Verification items for the finished model (mm, model axes). A direction names the side the tool comes from. Give positions to 0.01 mm unless a question says otherwise; leave off trailing zeros. Order: outer loops, then holes, each group sorted by start corner. A loop starts at its lowest first (then second) coordinate and runs counter-clockwise, first axis right, second up. Notation, with made-up numbers: (65, -35.5) - (77, -35.5) arc R19 cw to (77, -5.5) - close; hole circle Ø5 at (-19, 77). An arc over 180 degrees is marked (long way). Answer as a JSON object with one key per item and string values.
```python
from build123d import *

# Parameters (mm, degrees)
SKETCH_1_W          = 34
SKETCH_1_H          = 20
SKETCH_1_W_2        = 3
SKETCH_1_H_2        = 12
SKETCH_1_W_3        = 10
SKETCH_1_H_3        = 3
EXTRUDE_1_DEPTH     = 3
SKETCH_2_W          = 2.8
SKETCH_2_H          = 3.3
SKETCH_2_W_2        = 3.2
SKETCH_2_H_2        = 1.35
SKETCH_2_W_3        = 6
CUT_EXTRUDE_1_DEPTH = 3
SKETCH_4_W          = 20
SKETCH_4_H          = 20
SKETCH_4_W_2        = 10
SKETCH_4_H_2        = 3
EXTRUDE_2_DEPTH     = 3
SKETCH_5_W          = 3.2
SKETCH_5_H          = 2.8
SKETCH_5_W_2        = 1.4
SKETCH_5_H_2        = 3.2
SKETCH_5_H_3        = 6
SKETCH_5_W_3        = 1.35
SKETCH_5_W_4        = 3.3
CUT_EXTRUDE_2_DEPTH = 3


with BuildPart() as part:
    # 草图1 → 凸台-拉伸1 (new body)
    with BuildSketch(Plane(origin=(0, 0, 0), x_dir=(1, 0, 0), z_dir=(0, 1, 0))):
        Rectangle(SKETCH_1_W, SKETCH_1_H)
        with Locations((18.5, 0)):
            Rectangle(SKETCH_1_W_2, SKETCH_1_H_2)
        with Locations((0, 11.5)):
            Rectangle(SKETCH_1_W_3, SKETCH_1_H_3)
        with Locations((0, -11.5)):
            Rectangle(SKETCH_1_W_3, SKETCH_1_H_3)
    extrude(amount=EXTRUDE_1_DEPTH)

    # 草图2 → 切除-拉伸1 (cut)
    with BuildSketch(Plane(origin=(0, 3, 0), x_dir=(1, 0, 0), z_dir=(0, 1, 0))):
        with Locations((9.4, 0)):
            Rectangle(SKETCH_2_W, SKETCH_2_H)
        with Locations((12.4, 2.325)):
            Rectangle(SKETCH_2_W_2, SKETCH_2_H_2)
        with Locations((12.4, 0)):
            Rectangle(SKETCH_2_W_2, SKETCH_2_H)
        with Locations((12.4, -2.325)):
            Rectangle(SKETCH_2_W_2, SKETCH_2_H_2)
        with Locations((17, 0)):
            Rectangle(SKETCH_2_W_3, SKETCH_2_H)
    extrude(amount=-CUT_EXTRUDE_1_DEPTH, mode=Mode.SUBTRACT)

    # 草图4 → 凸台-拉伸2 (add)
    with BuildSketch(Plane(origin=(0, 3, 0), x_dir=(1, 0, 0), z_dir=(0, 1, 0))):
        with Locations((-27, 0)):
            Rectangle(SKETCH_4_W, SKETCH_4_H)
        with Locations((-24.6, 11.5)):
            Rectangle(SKETCH_4_W_2, SKETCH_4_H_2)
        with Locations((-24.6, -11.5)):
            Rectangle(SKETCH_4_W_2, SKETCH_4_H_2)
    extrude(amount=-EXTRUDE_2_DEPTH)

    # 草图5 → 切除-拉伸2 (cut)
    with BuildSketch(Plane(origin=(0, 3, 0), x_dir=(1, 0, 0), z_dir=(0, 1, 0))):
        with Locations((0, 2.4)):
            Rectangle(SKETCH_5_W, SKETCH_5_H)
        with Locations((-2.3, 5.4)):
            Rectangle(SKETCH_5_W_2, SKETCH_5_H_2)
        with Locations((0, 10)):
            Rectangle(SKETCH_5_W, SKETCH_5_H_3)
        with Locations((0, 5.4)):
            Rectangle(SKETCH_5_W, SKETCH_5_H_2)
        with Locations((2.3, 5.4)):
            Rectangle(SKETCH_5_W_2, SKETCH_5_H_2)
        with Locations((-26.925, -5.4)):
            Rectangle(SKETCH_5_W_3, SKETCH_5_H_2)
        with Locations((-24.6, -2.4)):
            Rectangle(SKETCH_5_W_4, SKETCH_5_H)
        with Locations((-22.275, -5.4)):
            Rectangle(SKETCH_5_W_3, SKETCH_5_H_2)
        with Locations((-24.6, -5.4)):
            Rectangle(SKETCH_5_W_4, SKETCH_5_H_2)
        with Locations((-24.6, -10)):
            Rectangle(SKETCH_5_W_4, SKETCH_5_H_3)
    extrude(amount=-CUT_EXTRUDE_2_DEPTH, mode=Mode.SUBTRACT)


solid = part.part
```
(1) Access from +Z, -Z, +X, -X, +Y, -Y to the whole of each face (thin tool, end or side, straight path). Record for faces 5 (the flat face through (-33, 2, -10)), 6 (the flat face through (11, 1, 10)), 7 (the flat face through (-19.6, 2, 12)), 8 (the flat face through (10.8, 2, 2)).
Computed values:
{"face 5": "-Z, -X, +Y, -Y", "face 6": "+Z, +X, +Y, -Y", "face 7": "+Z, +Y, -Y", "face 8": "+Y, -Y"}
(2) Release check for a two-part mould opening along Z. For faces 1 (the flat face through (10.8, 2, -2)), 2 (the flat face through (-28, 2, 13)), 3 (the flat face through (1.6, 2, -2)), 4 (the flat face through (-3, 1, -13)) record: pulls with the +Z half, pulls with the -Z half, needs draft (parallel to the pull), parting line crosses it, or undercut.
Computed values:
{"face 1": "undercut", "face 2": "pulls with the +Z half", "face 3": "needs draft", "face 4": "pulls with the -Z half"}
(3) Section check A-A (z = -9). Record the cut outline in (x, y).
Computed values:
{"outline": "(-37, 0) - (-1.6, 0) - (-1.6, 3) - (-37, 3) - close; (1.6, 0) - (17, 0) - (17, 3) - (1.6, 3) - close"}
(4) Material ranges on line 1 along X through (y, z) = (1.05, 2.25); line 2 along X through (y, z) = (0.7, 10.75); line 3 along X through (y, z) = (1.15, 3.25), recorded low to high. Write a range as [from, to].
Computed values:
{"line 1": "x = [-37, -26.25], [-22.95, 10.8], [14, 20]", "line 2": "x = [-29.6, -26.25], [-22.95, -19.6], [-5, 5]", "line 3": "x = [-37, -26.25], [-22.95, 20]"}
(5) Section check B-B (x = 0.5). Record the cut outline in (y, z), then the cut area to 3 significant figures.
Computed values:
{"outline": "(0, -1) - (3, -1) - (3, 13) - (0, 13) - close", "area": "42.0 mm²"}
(6) Gauge pin test, flat ends, axial feed: pin 1 Ø5 at (x, z) = (-30.5, 8.5) entering from -Y; pin 2 Ø1.5 at (y, z) = (1.5, 11) entering from +X; pin 3 Ø1.5 at (y, z) = (1.5, 7) entering from +X; pin 4 Ø1.5 at (x, y) = (12, 1.5) entering from +Z. Record the tip position at first contact, or that the pin passes through.
Computed values:
{"pin 1": "stops at y = 0", "pin 2": "stops at x = 5", "pin 3": "stops at x = 17", "pin 4": "stops at z = 10"}
(7) Section check C-C (x = -7.5). Record the cut outline in (y, z), then the cut area to 3 significant figures.
Computed values:
{"outline": "(0, -10) - (3, -10) - (3, 10) - (0, 10) - close", "area": "60.0 mm²"}
